Input: part model. Units: mm. Frame: model coordinates. Face numbers are marked on the shaded views. A direction names the side the tool comes from. Round coordinates to 2 decimals unless told otherwise and drop trailing zeros. Loops run counter-clockwise (first coordinate to the right, second up) from the corner with the lowest first, then second, coordinate; pieces in that order, holes last. Notation, with made-up numbers: (-24, 55) -> (-14, 55) arc R23 cw to (-14, 87) -> close; hole circle Ø7 at (2, -36). An arc over 180 degrees is marked (long way). Answer in a Markdown table with one row per item. Add a question column.
Q1. Pin query (flat end, axial travel): pin 1 (4 mm diameter, centred on x = 0.5, z = -7.5, fed in from -Y); pin 2 (2 mm diameter, centred on y = 6, z = -3, fed in from -X); pin 3 (1 mm diameter, centred on x = 6.5, y = 2.5, fed in from -Z); pin 4 (4 mm diameter, centred on y = 2, z = 3, fed in from -X). Return the tip coordinate at first contact, or that it passes through.
Q2. Section D-D, the plane z = 7.25. Output: boundary loops of the cut face in (x, y), and give its area (3 significant figures).
Q3. Mould query, pull axis Z, two halves, no side actions, for the marked faces 1, 2 and 3. Classes: pulls with the +Z half, pulls with the -Z half, needs draft (parallel to the pull), parting line crosses it, or undercut.
Q4. Ray query, L1, parallel to X at y = 1.9, z = 0; L2, parallel to Z at x = -4.25, y = 2.55; L3, parallel to X at y = 7, z = 0. Return the intervals inside material, ascending. Write a range as from..to.
Q5. Section B-B, the plane x = -4.25. Output: boundary loops of the cut face in (y, z).
Q6. Section C-C, the plane y = 6.25. Output: boundary loops of the cut face in (x, z), and give its area (3 significant figures).
Q7. Section A-A, the plane z = 0. Output: boundary loops of the cut face in (x, y).
Q8. Reachability of the marked faces 4 and 5 from +Z, -Z, +X, -X, +Y, -Y: full face, straight path, thin tool, end or side. Return the list, or none.
```python
from build123d import *

# Parameters (mm, degrees)
SKETCH1_R           = 8
BOSS_EXTRUDE1_DEPTH = 8
SKETCH2_R           = 8.214701508
SKETCH2_R_2         = 4.5
BOSS_EXTRUDE2_DEPTH = 3


with BuildPart() as part:
    # Sketch1 → Boss-Extrude1 (new body)
    with BuildSketch(Plane(origin=(0, 0, 0), x_dir=(1, 0, 0), z_dir=(0, 1, 0))):
        with BuildLine():
            Line((-5.15, 11.1), (5.15, 11.1))
            ThreePointArc((5.15, 11.1), (16.25, 0), (5.15, -11.1))
            Line((5.15, -11.1), (-5.15, -11.1))
            ThreePointArc((-5.15, -11.1), (-16.25, 0), (-5.15, 11.1))
        make_face()
        with Locations(Location((-4.25, 0, 0), (0, 0, 270))):
            Circle(SKETCH1_R, mode=Mode.SUBTRACT)
    extrude(amount=BOSS_EXTRUDE1_DEPTH)

    # Sketch2 → Boss-Extrude2 (add)
    with BuildSketch(Plane(origin=(0, 8, 0), x_dir=(1, 0, 0), z_dir=(0, 1, 0))):
        with Locations((-4.25, 0)):
            Circle(SKETCH2_R)
        with Locations(Location((-4.25, 0, 0), (0, 0, 270))):
            Circle(SKETCH2_R_2, mode=Mode.SUBTRACT)
    extrude(amount=-BOSS_EXTRUDE2_DEPTH)


solid = part.part
```
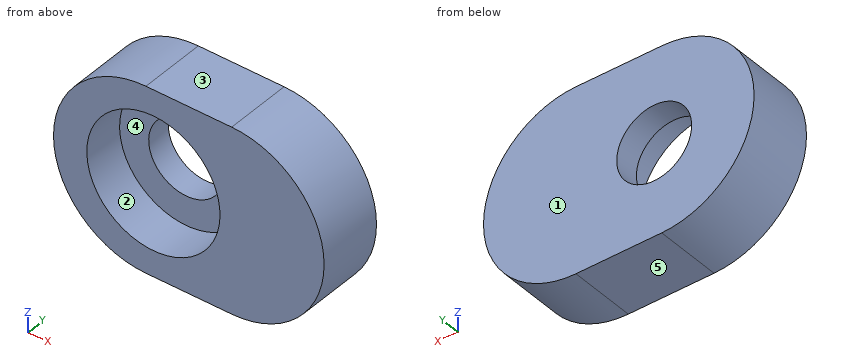
Answer block:
| question | item | result |
|---|---|---|
| 1 | pin 1 | y = 0 |
| 1 | pin 2 | x = -16.07 |
| 1 | pin 3 | z = -11.07 |
| 1 | pin 4 | x = -16.2 |
| 2 | outline | (-13.56, 0) -> (-7.63, 0) -> (-7.63, 5) -> (-0.87, 5) -> (-0.87, 0) -> (13.56, 0) -> (13.56, 8) -> (-13.56, 8) -> close |
| 2 | area | 183 mm^2 |
| 3 | face 1 | needs draft |
| 3 | face 2 | undercut |
| 3 | face 3 | pulls with the +Z half |
| 4 | L1 | -16.25..-12.25, 3.75..16.25 |
| 4 | L2 | -11.1..-8, 8..11.1 |
| 4 | L3 | -16.25..-8.75, 0.25..16.25 |
| 5 | outline | (0, -11.1) -> (8, -11.1) -> (8, -4.5) -> (5, -4.5) -> (5, -8) -> (0, -8) -> close; (0, 8) -> (5, 8) -> (5, 4.5) -> (8, 4.5) -> (8, 11.1) -> (0, 11.1) -> close |
| 6 | outline | (-5.15, -11.1) -> (5.15, -11.1) arc R11.1 ccw to (5.15, 11.1) -> (-5.15, 11.1) arc R11.1 ccw to start; hole circle Ø9 at (-4.25, 0) |
| 6 | area | 552 mm^2 |
| 7 | outline | (-16.25, 0) -> (-12.25, 0) -> (-12.25, 5) -> (-8.75, 5) -> (-8.75, 8) -> (-16.25, 8) -> close; (0.25, 5) -> (3.75, 5) -> (3.75, 0) -> (16.25, 0) -> (16.25, 8) -> (0.25, 8) -> close |
| 8 | face 4 | -Y |
| 8 | face 5 | -Z, +X, -X, +Y, -Y |
